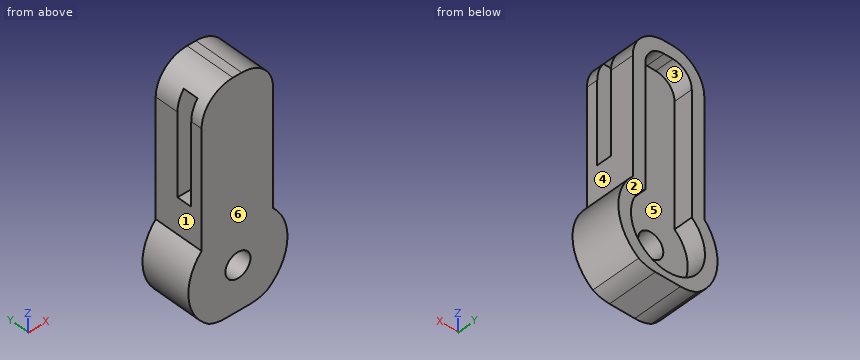
```python
from build123d import *

# Parameters (mm, degrees)
SKETCH_1_W          = 8
SKETCH_1_H          = 18
EXTRUDE_1_DEPTH     = 4
CUT_EXTRUDE_4_DEPTH = 1.5
SKETCH_6_W          = 8
SKETCH_6_H          = 1.2
CUT_EXTRUDE_5_DEPTH = 13.68857754
SKETCH_7_R          = 1
CUT_EXTRUDE_6_DEPTH = 11.161200716
FILLET_1_R          = 3
FILLET_2_R          = 2
FILLET_3_R          = 1.5
CUT_EXTRUDE_START   = -4
CUT_EXTRUDE_7_DEPTH = 4


# Read off the part's stored shape, not the designer's step: 切除-拉伸7
with BuildPart() as part:
    # 草图1 → 凸台-拉伸1 (new body)
    with BuildSketch(Plane(origin=(0, 0, 0), x_dir=(1, 0, 0), z_dir=(0, 1, 0))):
        Rectangle(SKETCH_1_W, SKETCH_1_H)
    extrude(amount=EXTRUDE_1_DEPTH)

    # 草图5 → 切除-拉伸4 (cut)
    with BuildSketch(Plane(origin=(0, 4, 0), x_dir=(1, 0, 0), z_dir=(0, 1, 0))):
        with BuildLine():
            Line((1.802116427, -8), (-1.897883573, -8))
            Line((-1.897883573, -8), (-1.897883573, 3.241562942))
            ThreePointArc((-1.897883573, 3.241562942), (0.061482678, 8.449359232), (1.802116427, 3.164432321))
            Line((1.802116427, 3.164432321), (1.802116427, -8))
        make_face()
    extrude(amount=-CUT_EXTRUDE_4_DEPTH, mode=Mode.SUBTRACT)

    # 草图6 → 切除-拉伸5 (cut, through all)
    with BuildSketch(Plane(origin=(4, 0, 0), x_dir=(0, 0, -1), z_dir=(1, 0, 0))):
        with Locations((-4, 1.5)):
            Rectangle(SKETCH_6_W, SKETCH_6_H)
    extrude(amount=-CUT_EXTRUDE_5_DEPTH, mode=Mode.SUBTRACT)

    # 草图7 → 切除-拉伸6 (cut, through all)
    with BuildSketch(Plane(origin=(0, 2.5, 0), x_dir=(1, 0, 0), z_dir=(0, 1, 0))):
        with Locations(Location((0, 5.5, 0), (0, 0, 270))):
            Circle(SKETCH_7_R)
    extrude(amount=-CUT_EXTRUDE_6_DEPTH, mode=Mode.SUBTRACT)

    # 圆角1
    fillet_1_edges = [part.edges().sort_by_distance(p)[0] for p in [
        (-4, 2, -9),
        (4, 2, -9),
    ]]
    fillet(fillet_1_edges, radius=FILLET_1_R)

    # 圆角2
    # the kernel refuses this fillet: 2 mm, written as the material it takes off along each edge
    with BuildSketch(Plane(origin=(4, -5, 9), x_dir=(0, 0, -1), z_dir=(0, 1, 0)), Plane(origin=(-4, -5, 9), x_dir=(1, 0, 0), z_dir=(0, 1, 0))) as fillet_2_piece_1:
        with BuildLine():
            CenterArc((FILLET_2_R, FILLET_2_R), FILLET_2_R, 180, 90)
            Line((0, FILLET_2_R), (0, 0))
            Line((0, 0), (FILLET_2_R, 0))
        make_face()
    extrude(amount=14, mode=Mode.SUBTRACT)

    # 圆角3
    fillet_3_edges = [part.edges().sort_by_distance(p)[0] for p in [
        (1.802116427, 3.25, 8),
        (-1.897883573, 3.25, 8),
    ]]
    fillet(fillet_3_edges, radius=FILLET_3_R)

    # 切除-拉伸7 outline → 切除-拉伸7 (cut)
    with BuildSketch(Plane(origin=(0, 4, 0), x_dir=(1, 0, 0), z_dir=(0, 1, 0)).offset(CUT_EXTRUDE_START)):
        with BuildLine():
            ThreePointArc((-2.897883573, 2.815829589), (-3.931803195, 5.878713127), (-2.332278942, 8.687942116))
            ThreePointArc((-2.332278942, 8.687942116), (-3.549199564, 7.581638893), (-4, 6))
            Line((-4, 6), (-4, -7))
            ThreePointArc((-4, -7), (-3.414213562, -8.414213562), (-2, -9))
            Line((-2, -9), (-0.397883573, -9))
            ThreePointArc((-0.397883573, -9), (-2.165650526, -8.267766953), (-2.897883573, -6.5))
            Line((-2.897883573, -6.5), (-2.897883573, 2.815829589))
        make_face()
        with BuildLine():
            Line((4, -7), (4, 6))
            ThreePointArc((4, 6), (3.549199564, 7.581638893), (2.332278942, 8.687942117))
            ThreePointArc((2.332278942, 8.687942117), (3.937831945, 5.809805707), (2.802116427, 2.71600224))
            Line((2.802116427, 2.71600224), (2.802116427, -6.5))
            ThreePointArc((2.802116427, -6.5), (2.06988338, -8.267766953), (0.302116427, -9))
            Line((0.302116427, -9), (2, -9))
            ThreePointArc((2, -9), (3.414213562, -8.414213562), (4, -7))
        make_face()
    extrude(amount=CUT_EXTRUDE_7_DEPTH, mode=Mode.SUBTRACT)


solid = part.part
```
Geometry check sheet. Reference: the model listing, model coordinates, mm. Face numbers are marked on the shaded views. A direction names the side the tool comes from. Coordinates: 2 decimals unless noted, no trailing zeros. Order: outer loops, then holes, each group sorted by start corner. A loop starts at its lowest first (then second) coordinate and runs counter-clockwise, first axis right, second up. Notation, with made-up numbers: (40.25, 9.5) - (93.25, 9.5) arc R31 ccw to (93.25, 34.5) - close; hole circle Ø4 at (8, 39.5). An arc over 180 degrees is marked (long way). Answer in a Markdown table with one row per item. Add a question column.
1. Section check B-B (x = 0). Enter the section's corners in (y, z), plus the area to 3 significant figures.
2. Access from +Z, -Z, +X, -X, +Y, -Y to the whole of each face (thin tool, end or side, straight path). Record for the marked faces 4, 5 and 6.
3. Section check D-D (z = -5.5). Enter the section's corners in (x, y).
4. Draft check along X on the marked faces 1, 2 and 3. Enter one of: +X half, -X half, draft (parallel to the pull), parting line (faces both ways), or undercut.
5. Section check C-C (y = 0.6). Enter the section's corners in (x, z), plus the area to 3 significant figures.
6. Section check A-A (y = 1.4). Enter the section's corners in (x, z).
7. Material ranges on L1, parallel to X at y = 3.7, z = -5.5; L2, parallel to Y at x = 0.5, z = 4; L3, parallel to Y at x = 1.75, z = -6.75, recorded low to high. Write a range as [from, to].
8. Gauge pin test, flat ends, axial feed: pin 1 Ø1.2 at (y, z) = (3, 0.5) entering from +X; pin 2 Ø3 at (x, z) = (0, -5.5) entering from +Y; pin 3 Ø1 at (x, y) = (-1, 1.5) entering from +Z. Record the tip position at first contact, or that the pin passes through.
Data:
| question | item | result |
|---|---|---|
| 1 | outline | (0, -9) - (4, -9) - (4, -8.45) - (2.5, -8.45) - (2.5, -6.5) - (0, -6.5) - close; (0, -4.5) - (2.5, -4.5) - (2.5, 8) - (4, 8) - (4, 9) - (0, 9) - close; hole (0.9, 0) - (2.1, 0) - (2.1, 8) - (0.9, 8) - close |
| 1 | area | 32.7 mm² |
| 2 | face 4 | +Z, +X, +Y, -Y |
| 2 | face 5 | +Y |
| 2 | face 6 | +Z, -Z, +X, -X, -Y |
| 3 | outline | (-3.95, 0) - (-1, 0) - (-1, 2.5) - (-2.95, 2.5) - (-2.95, 4) - (-3.95, 4) - close; (1, 0) - (3.95, 0) - (3.95, 4) - (2.95, 4) - (2.95, 2.5) - (1, 2.5) - close |
| 4 | face 1 | -X half |
| 4 | face 2 | draft |
| 4 | face 3 | undercut |
| 5 | outline | (-2.9, -2.82) arc R3.95 ccw to (-2.33, -8.69) arc R3 ccw to (-1, -9) - (1, -9) arc R3 ccw to (2.33, -8.69) arc R3.95 ccw to (2.8, -2.72) - (2.8, 6.5) arc R2.5 ccw to (0.3, 9) - (-0.4, 9) arc R2.5 ccw to (-2.9, 6.5) - close; hole circle Ø2 at (0, -5.5) |
| 5 | area | 104 mm² |
| 6 | outline | (-2.9, -2.82) arc R3.95 ccw to (-2.33, -8.69) arc R3 ccw to (-1, -9) - (1, -9) arc R3 ccw to (2.33, -8.69) arc R3.95 ccw to (2.8, -2.72) - (2.8, 0) - (-2.9, 0) - close; (-2.4, 8) - (2.3, 8) arc R2.5 ccw to (0.3, 9) - (-0.4, 9) arc R2.5 ccw to start; hole circle Ø2 at (0, -5.5) |
| 7 | L1 | x = [-3.95, -2.95], [2.95, 3.95] |
| 7 | L2 | y = [0, 0.9], [2.1, 2.5] |
| 7 | L3 | y = [0, 2.5] |
| 8 | pin 1 | stops at x = 2.8 |
| 8 | pin 2 | stops at y = 2.5 |
| 8 | pin 3 | stops at z = 9 |
